CAD build for the part. Positions are in the model's coordinates, mm. Give positions to 0.01 mm unless a question says otherwise; leave off trailing zeros. Loops run counter-clockwise (first coordinate to the right, second up) from the corner with the lowest first, then second, coordinate; pieces in that order, holes last.
Item 1: Probe probe 1 along X at (y, z) = (-41.5, 0); probe 2 along Z at (x, y) = (-2.5, -87). List the from-to ranges inside material, lowest first.
Item 2: Drop flat-ended pins along their axis: P1, Ø12, axis at x = 8.5, y = -16, coming from the -Z side; P2, Ø1, axis at y = -32.5, z = 1, coming from the +X side; P3, Ø3, axis at y = -13.5, z = 39.5, coming from the -X side. Give the stop position or say it passes through.
Item 3: Saw through at A-A on y = -50. Give the cut face in (x, z), plus the area to 3 significant figures.
from build123d import *

# Parameters (mm, degrees)
F1_DEPTH = 98.21704
F2_R     = 5.08
F4_R     = 5.08


# Not quite as in the source:
# - a fillet or chamfer that OpenCascade refuses, or shapes differently, is made with other operations: its cross-section is extruded or revolved along the edge and cut away or added


with BuildPart() as f1:
    # F0 (on Front) → F1 (new body)
    with BuildSketch(Plane.XZ):
        with BuildLine():
            ThreePointArc((11.7319880136, 49.2156378568), (-39.7076464503, -31.3547662371), (50.5946494444, 0))
            ThreePointArc((50.5946494444, 0), (39.7076464503, 31.3547662371), (11.7319880136, 49.2156378568))
        make_face()
        with BuildLine():
            ThreePointArc((44.2446494444, 0), (-34.7240452646, -27.4195128498), (10.2595373749, 43.0387139366))
            ThreePointArc((10.2595373749, 43.0387139366), (34.7240452646, 27.4195128498), (44.2446494444, 0))
        make_face(mode=Mode.SUBTRACT)
    extrude(amount=F1_DEPTH)

    # F2
    f2_edges = [f1.edges().sort_by_distance(p)[0] for p in [
        (-10.259537, -98.21704, -43.038714),
    ]]
    fillet(f2_edges, radius=F2_R)

    # F3: fillet of radius 5.08 on 1 edges, made by hand

    # F3_s1 → F3_t2 (revolve, cut)
    with BuildSketch(Plane.XY):
        with BuildLine():
            ThreePointArc((49.3246494444, -98.21704), (50.2665543256, -96.6529870592), (50.5946494444, -94.8569358349))
            Line((50.5946494444, -94.8569358349), (50.5946494444, -98.21704))
            Line((50.5946494444, -98.21704), (49.3246494444, -98.21704))
        make_face()
    revolve(axis=Axis((0, -98.21704, 0), (0, 1, 0)), mode=Mode.SUBTRACT)

    # F4
    f4_edges = [f1.edges().sort_by_distance(p)[0] for p in [
        (-10.259537, 0, -43.038714),
    ]]
    fillet(f4_edges, radius=F4_R)

    # F5: fillet of radius 5.08 on 1 edges, made by hand

    # F5_s1 → F5_t2 (revolve, cut)
    with BuildSketch(Plane.XY):
        with BuildLine():
            ThreePointArc((49.3246494444, 0), (50.2665543256, -1.5640529408), (50.5946494444, -3.3601041651))
            Line((50.5946494444, -3.3601041651), (50.5946494444, 0))
            Line((50.5946494444, 0), (49.3246494444, 0))
        make_face()
    revolve(axis=Axis((0, 0, 0), (0, -1, 0)), mode=Mode.SUBTRACT)


solid = f1.part
Results below:
1. probe 1: x = -50.59 to -44.24, 44.24 to 50.59
1. probe 2: z = -50.53 to -44.17, 44.17 to 50.53
2. P1: stops at z = -50.53
2. P2: stops at x = 50.59
2. P3: stops at x = -33.4
3. outline: circle Ø101.19 at (0, 0); hole circle Ø88.49 at (0, 0)
3. area: 1,890 mm2
